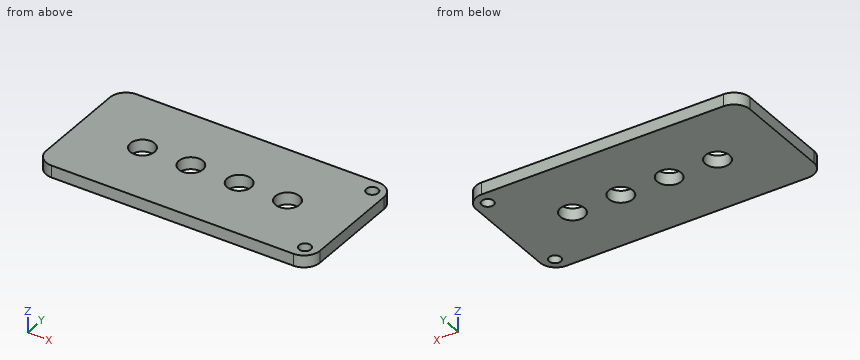
```python
from build123d import *

# Parameters (mm, degrees)
F0_R     = 2.38125
F0_R_2   = 1.1684
F1_DEPTH = 2.3622


with BuildPart() as f1:
    # F0 (on Top) → F1 (new body)
    with BuildSketch(Plane.XY):
        with BuildLine():
            ThreePointArc((27.001965, 9.530442), (26.072029, 11.775506), (23.826965, 12.705442))
            Line((23.826965, 12.705442), (-23.798035, 12.705442))
            ThreePointArc((-23.798035, 12.705442), (-26.043099, 11.775506), (-26.973035, 9.530442))
            Line((-26.973035, 9.530442), (-26.973035, -9.519558))
            ThreePointArc((-26.973035, -9.519558), (-26.043099, -11.764622), (-23.798035, -12.694558))
            Line((-23.798035, -12.694558), (23.826965, -12.694558))
            ThreePointArc((23.826965, -12.694558), (26.072029, -11.764622), (27.001965, -9.519558))
            Line((27.001965, -9.519558), (27.001965, 9.530442))
        make_face()
        with Locations((-14.273035, 0.005442)):
            Circle(F0_R, mode=Mode.SUBTRACT)
        with Locations((-4.748035, 0.005442)):
            Circle(F0_R, mode=Mode.SUBTRACT)
        with Locations((24.38142, -10.050331)):
            Circle(F0_R_2, mode=Mode.SUBTRACT)
        with Locations((4.776965, 0.005442)):
            Circle(F0_R, mode=Mode.SUBTRACT)
        with Locations((14.301965, 0.005442)):
            Circle(F0_R, mode=Mode.SUBTRACT)
        with Locations((24.38142, 10.050331)):
            Circle(F0_R_2, mode=Mode.SUBTRACT)
    extrude(amount=F1_DEPTH)


solid = f1.part
```
Source: CAD feature listing. Evaluate the final solid. Frame: model axes, mm. Round coordinates to 2 decimals unless told otherwise and drop trailing zeros. Write each loop counter-clockwise with the first axis right and the second up, starting at its lowest first coordinate (ties: lowest second). Pieces come first, ordered by that corner, then holes. Notation, with made-up numbers: M 35.5,-11.75 L 83.5,-11.75 A23 cw 83.5,10.25 Z; hole C 60.5,-3 d9. An arc over 180 degrees is marked long. Use CSV: the item, a comma, the result in double quotes. Start each with the question number.
Q1. Cut plane B-B on z = 0.65. Count the separate pieces of the cut face and the enclosed holes in it, plus the area to 3 significant figures.
Q2. Line query: line 1 (X direction, y = -1, z = 1.2); line 2 (X direction, y = 1.75, z = 1.4); line 3 (X direction, y = 10, z = 1.1). Output: solid intervals per line, ascending. Write a range as from..to.
Q3. Cut plane D-D on x = -6. Output: boundary loops of the cut face in (y, z), plus the area to 3 significant figures.
Q4. Cut plane C-C on y = -1.25. Output: boundary loops of the cut face in (x, z).
Q5. First-contact query: P1, Ø1.9, axis at x = 24.38, y = 10.05, coming from the +Z side. Flat tip, straight axial feed; report the tip coordinate or a pass-through.
Q6. Cut plane A-A on x = 12.5. Output: boundary loops of the cut face in (y, z), plus the area to 3 significant figures.
Results found:
1,separate pieces,"1"
1,enclosed holes,"6"
1,area,"1,280 mm^2"
2,line 1,"-26.97..-16.43, -12.11..-6.91, -2.59..2.62, 6.94..12.14, 16.46..27"
2,line 2,"-26.97..-15.89, -12.65..-6.37, -3.13..3.16, 6.4..12.68, 15.92..27"
2,line 3,"-26.94..23.21, 25.55..26.97"
3,outline,"M -12.69,0 L -2.02,0 L -2.02,2.36 L -12.69,2.36 Z; M 2.03,0 L 12.71,0 L 12.71,2.36 L 2.03,2.36 Z"
3,area,"50.4 mm^2"
4,outline,"M -26.97,0 L -16.3,0 L -16.3,2.36 L -26.97,2.36 Z; M -12.25,0 L -6.77,0 L -6.77,2.36 L -12.25,2.36 Z; M -2.72,0 L 2.75,0 L 2.75,2.36 L -2.72,2.36 Z; M 6.8,0 L 12.28,0 L 12.28,2.36 L 6.8,2.36 Z; M 16.33,0 L 27,0 L 27,2.36 L 16.33,2.36 Z"
5,P1,"through"
6,outline,"M -12.69,0 L -1.55,0 L -1.55,2.36 L -12.69,2.36 Z; M 1.56,0 L 12.71,0 L 12.71,2.36 L 1.56,2.36 Z"
6,area,"52.6 mm^2"
